Design review of the part built by this model. Coordinates are the model's own, in mm. Face numbers are marked on the shaded views. A direction names the side the tool comes from. Give positions to 0.01 mm unless a question says otherwise; leave off trailing zeros. Order: outer loops, then holes, each group sorted by start corner. A loop starts at its lowest first (then second) coordinate and runs counter-clockwise, first axis right, second up.
```python
from build123d import *

# Parameters (mm, degrees)
SKETCH_1_W          = 20
SKETCH_1_H          = 20
SKETCH_1_W_2        = 16
SKETCH_1_H_2        = 16
EXTRUDE_1_DEPTH     = 100
SKETCH_2_R          = 1.6
CUT_EXTRUDE_1_DEPTH = 104.923048454
SKETCH_3_R          = 1.6
CUT_EXTRUDE_2_DEPTH = 104.923048454


with BuildPart() as part:
    # 草图1 → 拉伸-薄壁1 (new body)
    with BuildSketch(Plane.XY):
        with Locations((10, 10)):
            Rectangle(SKETCH_1_W, SKETCH_1_H)
        with Locations((10, 10)):
            Rectangle(SKETCH_1_W_2, SKETCH_1_H_2, mode=Mode.SUBTRACT)
    extrude(amount=EXTRUDE_1_DEPTH)

    # 草图2 → 切除-拉伸1 (cut, through all)
    with BuildSketch(Plane.ZY):
        with Locations((10, 10)):
            Circle(SKETCH_2_R)
        with Locations((28, 10)):
            Circle(SKETCH_2_R)
    extrude(amount=-CUT_EXTRUDE_1_DEPTH, mode=Mode.SUBTRACT)

    # 草图3 → 切除-拉伸2 (cut, through all)
    with BuildSketch(Plane.ZY):
        with Locations((67.5, 10)):
            Circle(SKETCH_3_R)
        with Locations((40, 10)):
            Circle(SKETCH_3_R)
        with Locations((95, 10)):
            Circle(SKETCH_3_R)
    extrude(amount=-CUT_EXTRUDE_2_DEPTH, mode=Mode.SUBTRACT)


solid = part.part
```
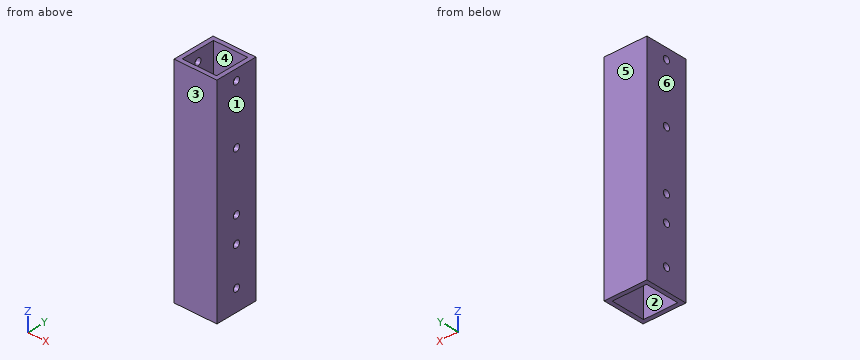
1. Draft analysis for pull direction Y (two halves, no side actions). For the marked faces 3, 4, 5 and 6, state which applies: pulls with the +Y half, pulls with the -Y half, needs draft (parallel to the pull), parting line crosses it, or undercut.
Recorded:
face 3: pulls with the -Y half
face 4: undercut
face 5: pulls with the +Y half
face 6: needs draft
2. For line 1 along Y through (x, z) = (8, 68.5); line 2 along Y through (x, z) = (1.5, 40), list the stretches that pass through material, from the lowest coordinate up.
Recorded:
line 1: y = 0 to 2, 18 to 20
line 2: y = 0 to 8.4, 11.6 to 20
3. Take a section at D-D (z = 40). State the section outline as (x, y) points, then the cut area to 3 significant figures.
Recorded:
outline: (0, 0) - (20, 0) - (20, 8.4) - (18, 8.4) - (18, 2) - (2, 2) - (2, 8.4) - (0, 8.4) - close; (0, 11.6) - (2, 11.6) - (2, 18) - (18, 18) - (18, 11.6) - (20, 11.6) - (20, 20) - (0, 20) - close
area: 131 mm2
4. Take a section at A-A (z = 51). State the section outline as (x, y) points, then the cut area to 3 significant figures.
Recorded:
outline: (0, 0) - (20, 0) - (20, 20) - (0, 20) - close; hole (2, 2) - (18, 2) - (18, 18) - (2, 18) - close
area: 144 mm2
5. Machinability: for the marked faces 1 and 2, which of the approach directions +Z, -Z, +X, -X, +Y, -Y give a long, thin tool a straight path to every point of the face, cutting with its end or side? Answer none if there is none.
Recorded:
face 1: +Z, -Z, +X, +Y, -Y
face 2: +Z, -Z
6. Take a section at B-B (y = 12.5). State the section outline as (x, z) points, then the cut area to 3 significant figures.
Recorded:
outline: (0, 0) - (2, 0) - (2, 100) - (0, 100) - close; (18, 0) - (20, 0) - (20, 100) - (18, 100) - close
area: 400 mm2
